Design review of the part built by this model. Coordinates are the model's own, in mm. Coordinates: 2 decimals unless noted, no trailing zeros. Loops run counter-clockwise (first coordinate to the right, second up) from the corner with the lowest first, then second, coordinate; pieces in that order, holes last. Notation, with made-up numbers: M 78,-13.5 L 122,-13.5 A14 ccw 122,10.5 Z; hole C -37,-6.75 d11. An arc over 180 degrees is marked long. Put each result on its own line as item: value. Start each with the question number.
(1) Take a section at B-B, the plane x = 2.5. Give the boundary of the cut face in (y, z), then the cut area to 3 significant figures.
(2) Clearance check with a flat-ended pin moving along its axis: pin 1 (5 mm diameter, centred on x = -3.5, z = 21.5, fed in from -Y). State where the tip first meets the part, or that it passes through.
(3) Take a section at C-C, the plane x = -1.75. Give the boundary of the cut face in (y, z).
(4) For probe 1 along Z at (x, y) = (0, 4.5); probe 2 along Y at (x, z) = (4.5, 23.5); probe 3 along Y at (x, z) = (2.25, 23.5), list the stretches that pass through material, from the lowest coordinate up. Write a range as [from, to].
(5) Take a section at A-A, the plane z = 26. Give the boundary of the cut face in (x, y).
```python
from build123d import *

# Parameters (mm, degrees)
BOSS_EXTRUDE1_DEPTH = 40.6146
SKETCH5_W           = 11.10345239
SKETCH5_H           = 12.145052052
SKETCH5_R           = 3.8481
CUT_EXTRUDE2_DEPTH  = 0.4445
SKETCH10_W          = 12.002544197
SKETCH10_H          = 11.794166694
SKETCH10_R          = 3.8481
CUT_EXTRUDE7_DEPTH  = 0.4445
SKETCH9_W           = 11.366817307
SKETCH9_H           = 11.947942936
SKETCH9_R           = 3.8481
CUT_EXTRUDE6_DEPTH  = 0.4445
SKETCH11_R          = 5.745102087
CUT_EXTRUDE8_DEPTH  = 4.9911


with BuildPart() as part:
    # Sketch1 → Boss-Extrude1 (new body)
    with BuildSketch(Plane.XY):
        Polygon((0, 5.499261314), (-4.7625, 2.749630657), (-4.7625, -2.749630657), (0, -5.499261314), (4.7625, -2.749630657), (4.7625, 2.749630657), align=None)
    extrude(amount=BOSS_EXTRUDE1_DEPTH)

    # Sketch5 → Cut-Extrude2 (cut, symmetric)
    with BuildSketch(Plane(origin=(0, 0, 22.6314), x_dir=(-1, 0, 0), z_dir=(0, 0, -1))):
        with Locations((-0.378227241, -0.09440181)):
            Rectangle(SKETCH5_W, SKETCH5_H)
        Circle(SKETCH5_R, mode=Mode.SUBTRACT)
    extrude(amount=CUT_EXTRUDE2_DEPTH, both=True, mode=Mode.SUBTRACT)

    # Sketch10 → Cut-Extrude7 (cut, symmetric)
    with BuildSketch(Plane(origin=(0, 0, 32.004), x_dir=(-1, 0, 0), z_dir=(0, 0, -1))):
        with Locations((-0.081621529, -0.253464989)):
            Rectangle(SKETCH10_W, SKETCH10_H)
        Circle(SKETCH10_R, mode=Mode.SUBTRACT)
    extrude(amount=CUT_EXTRUDE7_DEPTH, both=True, mode=Mode.SUBTRACT)

    # Sketch9 → Cut-Extrude6 (cut, symmetric)
    with BuildSketch(Plane.XY.offset(9.1059)):
        with Locations((0.130537015, 0.158516672)):
            Rectangle(SKETCH9_W, SKETCH9_H)
        Circle(SKETCH9_R, mode=Mode.SUBTRACT)
    extrude(amount=CUT_EXTRUDE6_DEPTH, both=True, mode=Mode.SUBTRACT)

    # Sketch11 → Cut-Extrude8 (cut)
    with BuildSketch(Plane.XY.offset(40.6146)):
        Circle(SKETCH11_R)
    extrude(amount=-CUT_EXTRUDE8_DEPTH, mode=Mode.SUBTRACT)


solid = part.part
```
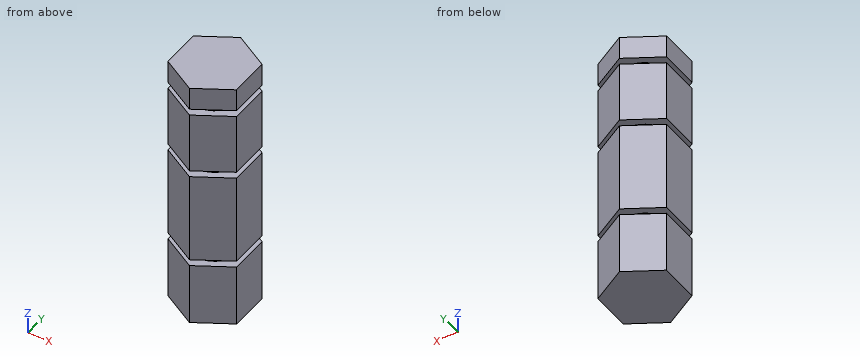
Computed values:
1. outline: M -4.06,0 L 4.06,0 L 4.06,8.66 L 2.93,8.66 L 2.93,9.55 L 4.06,9.55 L 4.06,22.19 L 2.93,22.19 L 2.93,23.08 L 4.06,23.08 L 4.06,31.56 L 2.93,31.56 L 2.93,32.45 L 4.06,32.45 L 4.06,35.62 L -4.06,35.62 L -4.06,32.45 L -2.93,32.45 L -2.93,31.56 L -4.06,31.56 L -4.06,23.08 L -2.93,23.08 L -2.93,22.19 L -4.06,22.19 L -4.06,9.55 L -2.93,9.55 L -2.93,8.66 L -4.06,8.66 Z
1. area: 283 mm^2
2. pin 1: stops at y = -4.92
3. outline: M -4.49,0 L 4.49,0 L 4.49,8.66 L 3.43,8.66 L 3.43,9.55 L 4.49,9.55 L 4.49,22.19 L 3.43,22.19 L 3.43,23.08 L 4.49,23.08 L 4.49,31.56 L 3.43,31.56 L 3.43,32.45 L 4.49,32.45 L 4.49,35.62 L -4.49,35.62 L -4.49,32.45 L -3.43,32.45 L -3.43,31.56 L -4.49,31.56 L -4.49,23.08 L -3.43,23.08 L -3.43,22.19 L -4.49,22.19 L -4.49,9.55 L -3.43,9.55 L -3.43,8.66 L -4.49,8.66 Z
4. probe 1: z = [0, 8.66], [9.55, 22.19], [23.08, 31.56], [32.45, 35.62]
4. probe 2: y = [-2.9, 2.9]
4. probe 3: y = [-4.2, 4.2]
5. outline: M -4.76,-2.75 L 0,-5.5 L 4.76,-2.75 L 4.76,2.75 L 0,5.5 L -4.76,2.75 Z
